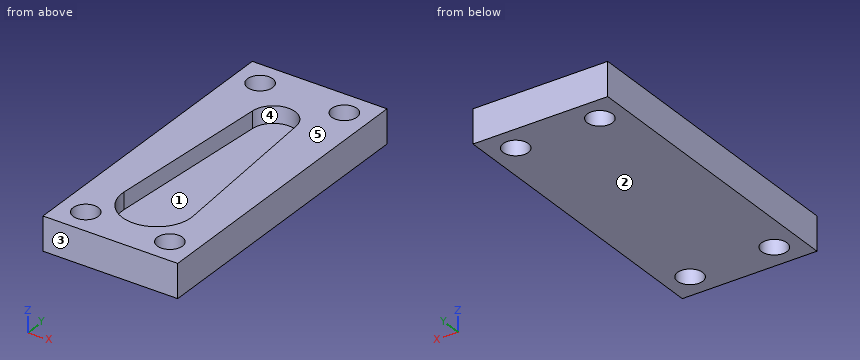
Autodesk Inventor part; units mm, degrees
ref_plane "YZ Plane" through (0, 0, 0) normal (1, 0, 0) x (0, 1, 0)
ref_plane "XZ Plane" through (0, 0, 0) normal (0, 1, 0) x (-1, 0, 0)
ref_plane "XY Plane" through (0, 0, 0) normal (0, 0, 1) x (1, 0, 0)
sketch "Sketch1" plane through (0, 0, 0) normal (0, 0, 1) x (1, 0, 0)
  line L0 (-12.7, 28.575) -> (12.7, 28.575)
  line L1 (12.7, 28.575) -> (12.7, -28.575)
  line L2 (12.7, -28.575) -> (-12.7, -28.575)
  line L3 (-12.7, -28.575) -> (-12.7, 28.575)
  point P0 (0, 0)
  point P1 (12.7, 0)
  point P2 (0, 28.575)
  dimension "d0" = 25.4
  dimension "d1" = 57.15
extrude "Extrusion1" add sketch "Sketch1" along normal blind 6.35
sketch "Sketch2" plane through (0, 0, 6.35) normal (0, 0, 1) x (1, 0, 0)
  arc A0 (-6.4964, -15.3835) -> (6.4964, -15.3835) centre (0, -15.875) ccw
  arc A1 (4.1031, 16.2496) -> (-4.1031, 16.2496) centre (0, 15.9392) ccw
  line L0 (4.1031, 16.2496) -> (6.4964, -15.3835)
  line L1 (-4.1031, 16.2496) -> (-6.4964, -15.3835)
  line L2 (-12.7, -28.575) -> (12.7, -28.575)
  line L3 (12.7, -28.575) -> (12.7, 28.575)
  dimension "d12" = 4.1148
  dimension "d13" = 6.515
  dimension "d18" = 4.327
  dimension "d23" = 12.7
  dimension "d54" = 31.8142
  dimension "d55" = 6.185
extrude "Extrusion2" cut sketch "Sketch2" against normal blind 3.175
sketch "Sketch4" plane through (0, 0, 6.35) normal (0, 0, 1) x (1, 0, 0)
  line L0 (7.9375, 23.8125) -> (-7.9375, 23.8125)
  line L1 (-7.9375, 23.8125) -> (-7.9375, -23.8125)
  line L2 (-7.9375, -23.8125) -> (7.9375, -23.8125)
  line L3 (7.9375, -23.8125) -> (7.9375, 23.8125)
  line L4 (12.7, 28.575) -> (12.7, -28.575)
  line L5 (-12.7, -28.575) -> (12.7, -28.575)
  point P0 (0, 0)
  dimension "d42" = 4.7625
  dimension "d43" = 4.7625
  dimension "d44" = 47.625
  dimension "d45" = 15.875
hole "Hole1" at (7.9375, 23.8125, 6.35) at (-7.9375, 23.8125, 6.35) at (-7.9375, -23.8125, 6.35) at (7.9375, -23.8125, 6.35) direction (0, 0, -1) diameter 4.7625 end through all
equation "\"d0\" = plate_width"
equation "\"d1\" = plate_height"
equation "\"d23\" = 0.5 * plate_width"
equation "\"d54\" = slot_centers"
equation "\"d42\" = hole_dist"
equation "\"d43\" = hole_dist"
equation "\"d44\" = plate_height - 2 * hole_dist"
equation "\"d45\" = plate_width - 2 * hole_dist"
equation "\"d46\" = hole_dia"
equation "\"plate_width\" = 25.4"
equation "\"plate_height\" = 57.15"
equation "\"slot_centers\" = 31.81417"
equation "\"hole_dia\" = 4.7625"
equation "\"hole_dist\" = 4.7625"
properties part number "ServoHornHolder"
Input: part model. Units: mm. Frame: model coordinates. Face numbers are marked on the shaded views. A direction names the side the tool comes from. Round coordinates to 2 decimals unless told otherwise and drop trailing zeros. Write each loop counter-clockwise with the first axis right and the second up, starting at its lowest first coordinate (ties: lowest second). Pieces come first, ordered by that corner, then holes. Notation, with made-up numbers: (-11, -12.75) -> (-5, -12.75) arc R15 cw to (-5, 1.25) -> close; hole circle Ø10 at (-10.5, -8). An arc over 180 degrees is marked (long way). Answer as CSV lines item,"result".
1. Section D-D (x = 0). Return the cut outline in (y, z) (3 decimals).
Geometry says:
outline,"(-28.575, 0) -> (28.575, 0) -> (28.575, 6.35) -> (20.054, 6.35) -> (20.054, 3.175) -> (-22.39, 3.175) -> (-22.39, 6.35) -> (-28.575, 6.35) -> close"
2. Mould query, pull axis Y, two halves, no side actions, for the marked faces 1, 2 and 3. Classes: +Y half, -Y half, draft (parallel to the pull), parting line (faces both ways), or undercut.
Geometry says:
face 1,"undercut"
face 2,"draft"
face 3,"-Y half"
3. Section C-C (y = -9.5). Return the cut outline in (x, z) (3 decimals), plus the area to 3 significant figures.
Geometry says:
outline,"(-12.7, 0) -> (12.7, 0) -> (12.7, 6.35) -> (6.051, 6.35) -> (6.051, 3.175) -> (-6.051, 3.175) -> (-6.051, 6.35) -> (-12.7, 6.35) -> close"
area,"123 mm^2"
4. Section B-B (z = 5). Return the cut outline in (x, y) (1 decimal).
Geometry says:
outline,"(-12.7, -28.6) -> (12.7, -28.6) -> (12.7, 28.6) -> (-12.7, 28.6) -> close; hole circle Ø4.8 at (-7.9, -23.8); hole circle Ø4.8 at (-7.9, 23.8); hole (-6.5, -15.4) arc R6.5 ccw (long way) to (6.5, -15.4) -> (4.1, 16.2) arc R4.1 ccw to (-4.1, 16.2) -> close; hole circle Ø4.8 at (7.9, -23.8); hole circle Ø4.8 at (7.9, 23.8)"
5. Reachability of the marked faces 4 and 5 from +Z, -Z, +X, -X, +Y, -Y: full face, straight path, thin tool, end or side. Return the list, or none.
Geometry says:
face 4,"+Z"
face 5,"+Z, +X, -X, +Y, -Y"
6. Ray query, L1, parallel to X at y = 26, z = 0.75; L2, parallel to X at y = -23.5, z = 4.75; L3, parallel to Y at x = 9, z = 1.25 (3 decimals). Return the intervals inside material, ascending. Write a range as [from, to].
Geometry says:
L1,"x = [-12.7, -8.88], [-7, 7], [8.88, 12.7]"
L2,"x = [-12.7, -10.3], [-5.58, 5.58], [10.3, 12.7]"
L3,"y = [-28.575, -25.944], [-21.681, 21.681], [25.944, 28.575]"
7. Section A-A (x = -9.75). Return the cut outline in (y, z) (3 decimals).
Geometry says:
outline,"(-28.575, 0) -> (-25.357, 0) -> (-25.357, 6.35) -> (-28.575, 6.35) -> close; (-22.268, 0) -> (22.268, 0) -> (22.268, 6.35) -> (-22.268, 6.35) -> close; (25.357, 0) -> (28.575, 0) -> (28.575, 6.35) -> (25.357, 6.35) -> close"
8. Contact query for a flat-ended pin moving along its axis: P1, Ø5.5, axis at x = -7.94, y = -23.81, coming from the +Z side. Output: stop coordinate, or through.
Geometry says:
P1,"stops at z = 6.35"
